Check sheet for the modelled part. Datum: model origin and axes. Units: mm. Give positions to 0.01 mm unless a question says otherwise; leave off trailing zeros. Order: outer loops, then holes, each group sorted by start corner. A loop starts at its lowest first (then second) coordinate and runs counter-clockwise, first axis right, second up. Notation, with made-up numbers: (-10, 63) - (47, 63) arc R11 ccw to (47, 81) - close; hole circle Ø11 at (-5, 48.5). An arc over 180 degrees is marked (long way). Answer in a Markdown table with one row per item.
from build123d import *

# Parameters (mm, degrees)
F0_R     = 50
F0_W     = 10
F0_H     = 20
F1_DEPTH = 5
F2_R     = 4.99999


# Not quite as in the source:
# - a fillet or chamfer is up to 0.001 mm smaller than in the source, because OpenCascade refuses the exact size


with BuildPart() as f1:
    # F0 (on Top) → F1 (new body)
    with BuildSketch(Plane.XY):
        Circle(F0_R)
        with Locations((0, 34)):
            Rectangle(F0_W, F0_H, mode=Mode.SUBTRACT)
    extrude(amount=F1_DEPTH)

    # F2 (radius 5 in the source; OpenCascade refuses exactly that, so slightly less here)
    f2_edges = [f1.edges().sort_by_distance(p)[0] for p in [
        (-50, 0, 5),
    ]]
    fillet(f2_edges, radius=F2_R)


solid = f1.part
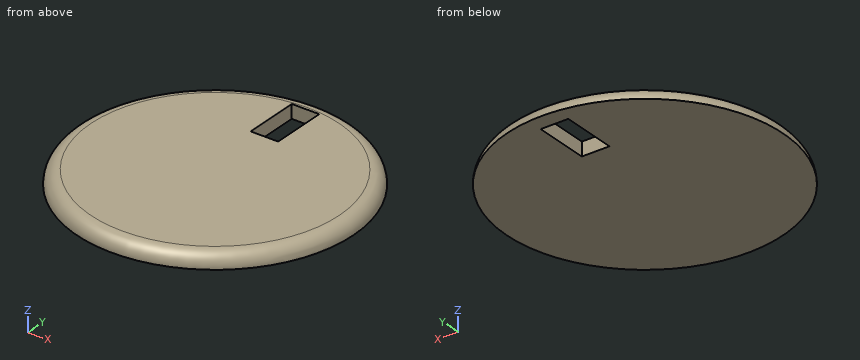
(1) Gauge pin test, flat ends, axial feed: P1, Ø1.5, axis at y = 29.5, z = 3.5, coming from the -X side; P2, Ø3, axis at x = -2, z = 2.5, coming from the -Y side; P3, Ø1.5, axis at y = 0, z = 1, coming from the -X side. Record the tip position at first contact, or that the pin passes through.
Geometry says:
| item | result |
|---|---|
| P1 | x = -39.55 |
| P2 | y = -49.86 |
| P3 | x = -49.99 |
(2) Cross-section at B-B, the plane z = 1.1. Record the cut outline in (x, y) (1 decimal).
Geometry says:
| item | result |
|---|---|
| outline | circle Ø99.8 at (0, 0); hole (-5, 24) - (5, 24) - (5, 44) - (-5, 44) - close |
(3) Thickness scan on L1, parallel to Y at x = 4, z = 3.45; L2, parallel to X at y = 35, z = 3.25; L3, parallel to Y at x = 25.5, z = 1.25. Record the ranges inside material, lowest first.
Geometry says:
| item | result |
|---|---|
| L1 | -48.45 to 24, 44 to 48.45 |
| L2 | -34.01 to -5, 5 to 34.01 |
| L3 | -42.82 to 42.82 |
